Input: part model. Units: mm. Frame: model coordinates. Give positions to 0.01 mm unless a question says otherwise; leave off trailing zeros. Order: outer loops, then holes, each group sorted by start corner. A loop starts at its lowest first (then second) coordinate and runs counter-clockwise, first axis right, second up.
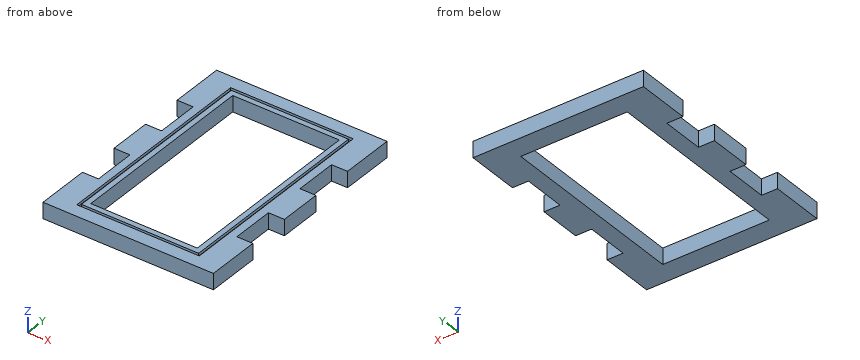
```python
from build123d import *

# Parameters (mm, degrees)
F0_W     = 127
F0_H     = 228.6
F1_DEPTH = 19.05
F2_W     = 146.05
F2_H     = 247.65
F2_W_2   = 139.7
F2_H_2   = 241.3
F3_DEPTH = 3.175


with BuildPart() as f1:
    # F0 (on Top) → F1 (new body)
    with BuildSketch(Plane.XY):
        Polygon((101.6, 139.7), (-101.6, 139.7), (-101.6, 76.2), (-82.55, 76.2), (-82.55, 25.4), (-101.6, 25.4), (-101.6, -25.4), (-82.55, -25.4), (-82.55, -76.2), (-101.6, -76.2), (-101.6, -139.7), (101.6, -139.7), (101.6, -76.2), (82.55, -76.2), (82.55, -25.4), (101.6, -25.4), (101.6, 25.4), (82.55, 25.4), (82.55, 76.2), (101.6, 76.2), align=None)
        Rectangle(F0_W, F0_H, mode=Mode.SUBTRACT)
    extrude(amount=F1_DEPTH)

    # F2 (on face) → F3 (cut)
    with BuildSketch(Plane.XY.offset(19.05)):
        Rectangle(F2_W, F2_H)
        Rectangle(F2_W_2, F2_H_2, mode=Mode.SUBTRACT)
    extrude(amount=-F3_DEPTH, mode=Mode.SUBTRACT)


solid = f1.part
```
1) Line query: probe 1 along X at (y, z) = (-76, 16.25) (3 decimals); probe 2 along Y at (x, z) = (50.5, 12.75); probe 3 along Y at (x, z) = (-89, 17.5). Output: solid intervals per line, ascending.
2) Cut plane A-A (x = 37). Return the cut outline in (y, z) (3 decimals), then the cut area to 3 significant figures.
3) Cut plane C-C (z = 11.25). Return the cut outline in (x, y), then the cut area to 3 significant figures.
4) Cut plane B-B (y = -73). Return the cut outline in (x, z) (3 decimals).
5) First-contact query: P1, Ø5.5, axis at y = 43.5, z = 8, coming from the -X side; P2, Ø2, axis at y = -58, z = 2.5, coming from the +X side; P3, Ø12, axis at x = -80, y = 109, coming from the -Z side. Flat tips, straight axial feed; report the tip coordinate or a pass-through.
Geometry says:
1. probe 1: x = -82.55 to -73.025, -69.85 to -63.5, 63.5 to 69.85, 73.025 to 82.55
1. probe 2: y = -139.7 to -114.3, 114.3 to 139.7
1. probe 3: y = -139.7 to -76.2, -25.4 to 25.4, 76.2 to 139.7
2. outline: (-139.7, 0) - (-114.3, 0) - (-114.3, 19.05) - (-120.65, 19.05) - (-120.65, 15.875) - (-123.825, 15.875) - (-123.825, 19.05) - (-139.7, 19.05) - close; (114.3, 0) - (139.7, 0) - (139.7, 19.05) - (123.825, 19.05) - (123.825, 15.875) - (120.65, 15.875) - (120.65, 19.05) - (114.3, 19.05) - close
2. area: 948 mm2
3. outline: (-101.6, -139.7) - (101.6, -139.7) - (101.6, -76.2) - (82.55, -76.2) - (82.55, -25.4) - (101.6, -25.4) - (101.6, 25.4) - (82.55, 25.4) - (82.55, 76.2) - (101.6, 76.2) - (101.6, 139.7) - (-101.6, 139.7) - (-101.6, 76.2) - (-82.55, 76.2) - (-82.55, 25.4) - (-101.6, 25.4) - (-101.6, -25.4) - (-82.55, -25.4) - (-82.55, -76.2) - (-101.6, -76.2) - close; hole (-63.5, -114.3) - (63.5, -114.3) - (63.5, 114.3) - (-63.5, 114.3) - close
3. area: 23,900 mm2
4. outline: (-82.55, 0) - (-63.5, 0) - (-63.5, 19.05) - (-69.85, 19.05) - (-69.85, 15.875) - (-73.025, 15.875) - (-73.025, 19.05) - (-82.55, 19.05) - close; (63.5, 0) - (82.55, 0) - (82.55, 19.05) - (73.025, 19.05) - (73.025, 15.875) - (69.85, 15.875) - (69.85, 19.05) - (63.5, 19.05) - close
5. P1: stops at x = -82.55
5. P2: stops at x = 82.55
5. P3: stops at z = 0
